```python
from build123d import *

# Parameters (mm, degrees)
SKETCH1_R                 = 15
BOSS_EXTRUDE1_DEPTH       = 7.5
BOSS_EXTRUDE2_START       = 13
SKETCH3_R                 = 7
SKETCH3_R_2               = 5
BOSS_EXTRUDE2_DEPTH       = 17
SKETCH3_4_R               = 3.5
SKETCH3_4_R_2             = 5
BOSS_EXTRUDE3_DEPTH       = 14
BOSS_EXTRUDE4_START       = 25
BOSS_EXTRUDE4_OUTLINE_R   = 5
BOSS_EXTRUDE4_OUTLINE_R_2 = 3.5
BOSS_EXTRUDE4_DEPTH       = 5
CIRPATTERN14_COUNT        = 3
CUT_EXTRUDE5_DEPTH        = 45.655518692


# Read off the part's stored shape, not the designer's step: Boss-Extrude4
with BuildPart() as part:
    # Sketch1 → Boss-Extrude1 (new, symmetric)
    with BuildSketch(Plane(origin=(0, 0, 0), x_dir=(1, 0, 0), z_dir=(0, 1, 0))):
        with Locations(Location((0, 0, 0), (0, 0, 270))):
            Circle(SKETCH1_R)
    extrude(amount=BOSS_EXTRUDE1_DEPTH, both=True)

    # Sketch3 → Boss-Extrude2 (add)
    with BuildSketch(Plane(origin=(0, 0, 0), x_dir=(0, 0, -1), z_dir=(1, 0, 0)).offset(BOSS_EXTRUDE2_START)):
        with Locations(Location((0, 0, 0), (0, 0, 180))):
            Circle(SKETCH3_R)
        with Locations(Location((0, 0, 0), (0, 0, 180))):
            Circle(SKETCH3_R_2, mode=Mode.SUBTRACT)
    boss_extrude2 = extrude(amount=BOSS_EXTRUDE2_DEPTH)

    # Sketch3<4> → Boss-Extrude3 (add)
    with BuildSketch(Plane(origin=(0, 0, 0), x_dir=(0, 0, -1), z_dir=(1, 0, 0))):
        Circle(SKETCH3_4_R)
        with Locations(Location((0, 0, 0), (0, 0, 180))):
            Circle(SKETCH3_4_R_2)
    boss_extrude3 = extrude(amount=BOSS_EXTRUDE3_DEPTH)

    # Boss-Extrude4 outline → Boss-Extrude4 (add)
    with BuildSketch(Plane(origin=(0, 0, 0), x_dir=(0, 0, -1), z_dir=(1, 0, 0)).offset(BOSS_EXTRUDE4_START)):
        Circle(BOSS_EXTRUDE4_OUTLINE_R)
        Circle(BOSS_EXTRUDE4_OUTLINE_R_2, mode=Mode.SUBTRACT)
    boss_extrude4 = extrude(amount=BOSS_EXTRUDE4_DEPTH)

    # CirPattern14: Boss-Extrude2, Boss-Extrude3, Boss-Extrude4 ×3 about axis
    cirpattern14_axis = Axis((0, -7.5, 0), (0, 1, 0))
    add([boss_extrude2.rotate(cirpattern14_axis, i * 360 / CIRPATTERN14_COUNT) for i in range(1, CIRPATTERN14_COUNT)])
    add([boss_extrude3.rotate(cirpattern14_axis, i * 360 / CIRPATTERN14_COUNT) for i in range(1, CIRPATTERN14_COUNT)])
    add([boss_extrude4.rotate(cirpattern14_axis, i * 360 / CIRPATTERN14_COUNT) for i in range(1, CIRPATTERN14_COUNT)])

    # Sketch4 → Cut-Extrude5 (cut, through all)
    with BuildSketch(Plane(origin=(0, 7.5, 0), x_dir=(1, 0, 0), z_dir=(0, 1, 0))):
        with BuildLine():
            ThreePointArc((5.864590062, 4.675102502), (5.315335108, 5.29123924), (4.701700296, 5.843287972))
            Line((4.701700296, 5.843287972), (2.968685581, 4.110273257))
            ThreePointArc((2.968685581, 4.110273257), (1.956146698, 4.677705679), (0.84109472, 5))
            Line((0.84109472, 5), (0.84109472, 7.452688084))
            ThreePointArc((0.84109472, 7.452688084), (0.017038352, 7.499980646), (-0.807224387, 7.456432712))
            Line((-0.807224387, 7.456432712), (-0.807224387, 5.005579798))
            ThreePointArc((-0.807224387, 5.005579798), (-1.924432811, 4.690842002), (-2.940790126, 4.130277686))
            Line((-2.940790126, 4.130277686), (-4.675102502, 5.864590062))
            ThreePointArc((-4.675102502, 5.864590062), (-5.29123924, 5.315335108), (-5.843287972, 4.701700296))
            Line((-5.843287972, 4.701700296), (-4.110273257, 2.968685581))
            ThreePointArc((-4.110273257, 2.968685581), (-4.677705679, 1.956146698), (-5, 0.84109472))
            Line((-5, 0.84109472), (-7.452688084, 0.84109472))
            ThreePointArc((-7.452688084, 0.84109472), (-7.499980646, 0.017038352), (-7.456432712, -0.807224387))
            Line((-7.456432712, -0.807224387), (-5.005579798, -0.807224387))
            ThreePointArc((-5.005579798, -0.807224387), (-4.690842002, -1.924432811), (-4.130277686, -2.940790126))
            Line((-4.130277686, -2.940790126), (-5.864590062, -4.675102502))
            ThreePointArc((-5.864590062, -4.675102502), (-5.315335108, -5.29123924), (-4.701700296, -5.843287972))
            Line((-4.701700296, -5.843287972), (-2.968685581, -4.110273257))
            ThreePointArc((-2.968685581, -4.110273257), (-1.956146698, -4.677705679), (-0.84109472, -5))
            Line((-0.84109472, -5), (-0.84109472, -7.452688084))
            ThreePointArc((-0.84109472, -7.452688084), (-0.017038352, -7.499980646), (0.807224387, -7.456432712))
            Line((0.807224387, -7.456432712), (0.807224387, -5.005579798))
            ThreePointArc((0.807224387, -5.005579798), (1.924432811, -4.690842002), (2.940790126, -4.130277686))
            Line((2.940790126, -4.130277686), (4.675102502, -5.864590062))
            ThreePointArc((4.675102502, -5.864590062), (5.29123924, -5.315335108), (5.843287972, -4.701700296))
            Line((5.843287972, -4.701700296), (4.110273257, -2.968685581))
            ThreePointArc((4.110273257, -2.968685581), (4.677705679, -1.956146698), (5, -0.84109472))
            Line((5, -0.84109472), (7.452688084, -0.84109472))
            ThreePointArc((7.452688084, -0.84109472), (7.499980646, -0.017038352), (7.456432712, 0.807224387))
            Line((7.456432712, 0.807224387), (5.005579798, 0.807224387))
            ThreePointArc((5.005579798, 0.807224387), (4.690842002, 1.924432811), (4.130277686, 2.940790126))
            Line((4.130277686, 2.940790126), (5.864590062, 4.675102502))
        make_face()
    extrude(amount=-CUT_EXTRUDE5_DEPTH, mode=Mode.SUBTRACT)


solid = part.part
```
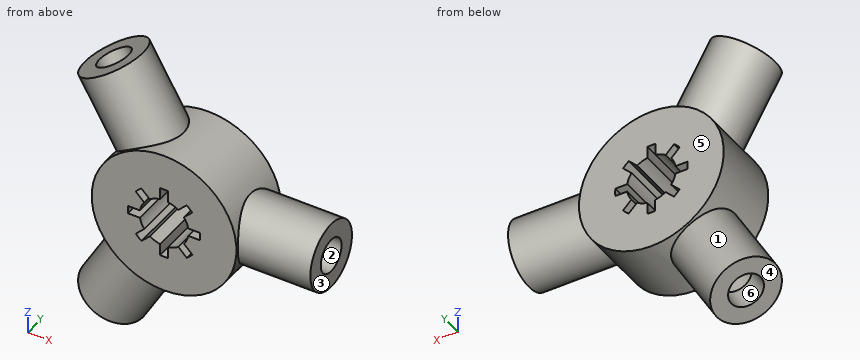
Can you work these out from the model? Positions are in its coordinate system, mm. Face numbers are marked on the shaded views. A direction names the side the tool comes from. Coordinates: 2 decimals unless noted, no trailing zeros. Loops run counter-clockwise (first coordinate to the right, second up) from the corner with the lowest first, then second, coordinate; pieces in that order, holes last. Notation, with made-up numbers: (-6.75, 79.25) -> (45.25, 79.25) arc R29 cw to (45.25, 115.25) -> close; hole circle Ø1 at (-13, 49). An arc over 180 degrees is marked (long way). Answer as a JSON object with one key per item and string values.
1) For the marked faces 1 and 2, which set-ups out of +Z, -Z, +X, -X, +Y, -Y let a thin tool reach every point of the face, with its end or its side?
Results:
{"face 1": "none", "face 2": "+X"}
2) Imagine slicing it at C-C (x = 19.5). Please give me the cut outline in (y, z).
Results:
{"outline": "circle Ø14 at (0, 0); hole circle Ø10 at (0, 0)"}
3) Imagine slicing it at B-B (x = 2). Please give me the cut outline in (y, z), then the cut area to 3 significant figures.
Results:
{"outline": "(-7.5, -14.87) -> (7.5, -14.87) -> (7.5, -4.66) -> (-7.5, -4.66) -> close; (-7.5, 4.66) -> (7.5, 4.66) -> (7.5, 14.87) -> (-7.5, 14.87) -> close", "area": "306 mm^2"}
4) Imagine slicing it at A-A (z = 0). Please give me the cut outline in (x, y).
Results:
{"outline": "(-15, -7.5) -> (-7.5, -7.5) -> (-7.5, 7.5) -> (-15, 7.5) -> close; (7.5, -7.5) -> (15, -7.5) -> (15, -7) -> (30, -7) -> (30, -3.5) -> (25, -3.5) -> (25, -5) -> (15, -5) -> (15, 5) -> (25, 5) -> (25, 3.5) -> (30, 3.5) -> (30, 7) -> (15, 7) -> (15, 7.5) -> (7.5, 7.5) -> close"}
5) If I drill on line 1 (Y direction, x = 19, z = 0); line 2 (Z direction, x = -4.5, y = 2); line 3 (Y direction, x = 26.1, z = 0), over which ranges is the centre line in solid material (lowest first)?
Results:
{"line 1": "y = -7 to -5, 5 to 7", "line 2": "z = -21.21 to -16.96, -14.31 to -5.69, -3.36 to -2.34, 2.34 to 3.31, 5.64 to 14.31, 16.96 to 21.21", "line 3": "y = -7 to -3.5, 3.5 to 7"}
6) Thinking about a two-plate mould opening in X: for the marked faces 3, 4, 5 and 6, which applies, pulls with the +X half, pulls with the -X half, needs draft (parallel to the pull), parting line crosses it, or undercut?
Results:
{"face 3": "pulls with the +X half", "face 4": "pulls with the -X half", "face 5": "needs draft", "face 6": "undercut"}
7) For P1, Ø5, axis at x = -4.5, y = -3.5, coming from the +Z side; P2, Ø10, axis at x = 6, z = 17, coming from the -Y side; P3, Ø2, axis at y = 2, z = 7, coming from the -X side; P4, Ø2.5, axis at x = -7, y = -2.5, coming from the +Z side, each with a flat end and sliding along its axis, tell me the tip position at first contact or that it passes through.
Results:
{"P1": "stops at z = 24.84", "P2": "stops at y = -7.5", "P3": "stops at x = -13.75", "P4": "stops at z = 27.53"}
